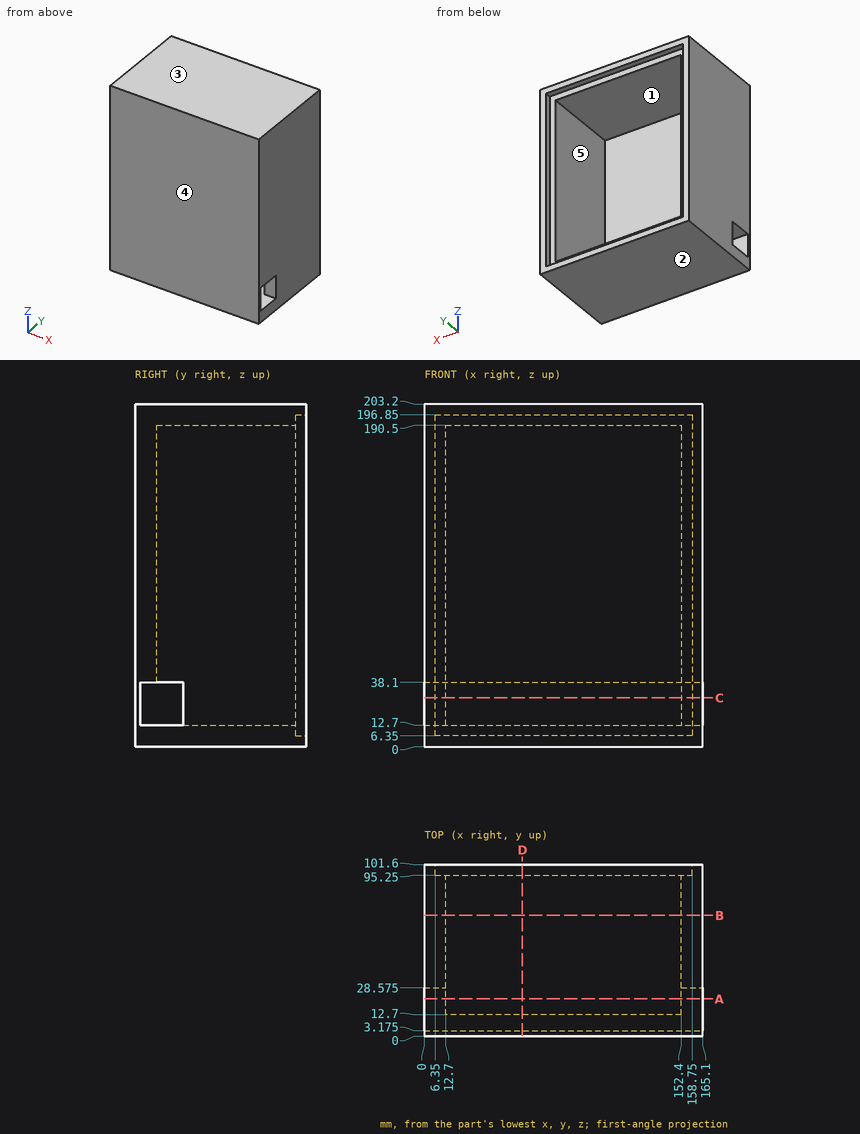
Design review of the part shown in the three views and the two pictorial views. Dimensions are in mm from the part's minimum x, y and z. A direction names the side the tool comes from. Give positions to 0.01 mm unless a question says otherwise; leave off trailing zeros. Write each loop counter-clockwise with the first axis right and the second up, starting at its lowest first coordinate (ties: lowest second). Pieces come first, ordered by that corner, then holes. Notation, with made-up numbers: (-0.5, 88.25) -> (35.5, 88.25) arc R25 ccw to (35.5, 107.25) -> close; hole circle Ø3 at (64, 53). An arc over 180 degrees is marked (long way). Answer in a Markdown table with one row per item.
1) For L1, parallel to X at y = 41.5, z = 89; L2, parallel to Z at x = 99.5, y = 73; L3, parallel to Y at x = 157.5, z = 17 (3 decimals), list the stretches that pass through material, from the lowest coordinate up. Write a range as [from, to].
Worked answers:
| item | result |
|---|---|
| L1 | [0, 12.7], [152.4, 165.1] |
| L2 | [0, 12.7], [190.5, 203.2] |
| L3 | [0, 3.175], [28.575, 95.25] |
2) Tool access review of the marked faces 4 and 5: name each direction out of +Z, -Z, +X, -X, +Y, -Y from which nothing blocks a thin tool from reaching the whole face with its end or side.
Worked answers:
| item | result |
|---|---|
| face 4 | +Z, -Z, +X, -X, -Y |
| face 5 | +Y |
3) Add section A-A on y = 22. State the section outline as (x, z) points, plus the area to 3 significant figures.
Worked answers:
| item | result |
|---|---|
| outline | (0, 0) -> (165.1, 0) -> (165.1, 12.7) -> (0, 12.7) -> close; (0, 38.1) -> (12.7, 38.1) -> (12.7, 190.5) -> (152.4, 190.5) -> (152.4, 38.1) -> (165.1, 38.1) -> (165.1, 203.2) -> (0, 203.2) -> close |
| area | 8,060 mm² |
4) Add section D-D on x = 58. State the section outline as (y, z) points (3 decimals), plus the area to 3 significant figures.
Worked answers:
| item | result |
|---|---|
| outline | (0, 0) -> (101.6, 0) -> (101.6, 6.35) -> (95.25, 6.35) -> (95.25, 12.7) -> (3.175, 12.7) -> (3.175, 38.1) -> (12.7, 38.1) -> (12.7, 190.5) -> (95.25, 190.5) -> (95.25, 196.85) -> (101.6, 196.85) -> (101.6, 203.2) -> (0, 203.2) -> close |
| area | 4,520 mm² |
5) Add section B-B on y = 71.5. State the section outline as (x, z) points, plus the area to 3 significant figures.
Worked answers:
| item | result |
|---|---|
| outline | (0, 0) -> (165.1, 0) -> (165.1, 203.2) -> (0, 203.2) -> close; hole (12.7, 12.7) -> (152.4, 12.7) -> (152.4, 190.5) -> (12.7, 190.5) -> close |
| area | 8,710 mm² |
6) Mouldability with a two-part tool opening along Z and no side actions: class the marked faces 1, 2 and 3 as +Z half, -Z half, draft (parallel to the pull), parting line (faces both ways), or undercut.
Worked answers:
| item | result |
|---|---|
| face 1 | undercut |
| face 2 | -Z half |
| face 3 | +Z half |
7) Clearance check with flat-ended pins moving along their axes: P1, Ø1, axis at x = 67.5, z = 33, coming from the +Y side (3 decimals); P2, Ø1, axis at x = 108, z = 140, coming from the +Y side; P3, Ø20.5, axis at x = 60, z = 22, coming from the +Y side. State where each tip first meets the part, or that it passes through.
Worked answers:
| item | result |
|---|---|
| P1 | y = 3.175 |
| P2 | y = 12.7 |
| P3 | y = 95.25 |
8) Add section C-C on z = 29. State the section outline as (x, y) points (3 decimals), plus the area to 3 significant figures.
Worked answers:
| item | result |
|---|---|
| outline | (0, 0) -> (165.1, 0) -> (165.1, 3.175) -> (0, 3.175) -> close; (0, 28.575) -> (12.7, 28.575) -> (12.7, 95.25) -> (6.35, 95.25) -> (6.35, 101.6) -> (0, 101.6) -> close; (152.4, 28.575) -> (165.1, 28.575) -> (165.1, 101.6) -> (158.75, 101.6) -> (158.75, 95.25) -> (152.4, 95.25) -> close |
| area | 2,300 mm² |
